Could you check a few things on this drawing? It's one solid part, dimensions in mm from its lowest x, y, z. Give positions to 0.01 mm unless a question says otherwise; leave off trailing zeros. Loops run counter-clockwise (first coordinate to the right, second up) from the corner with the lowest first, then second, coordinate; pieces in that order, holes last.
Q1. Suppose I cut it at B-B (x = 19.05). List the corners of the cut face in (y, z) for me, and give its area (3 significant figures).
Q2. Suppose I cut it at D-D (y = 43.9). List the corners of the cut face in (x, z) for me.
Q3. Suppose I cut it at C-C (z = 1.95). List the corners of the cut face in (x, y) for me, and give its area (3 significant figures).
Q4. Suppose I cut it at A-A (y = 25.4). List the corners of the cut face in (x, z) for me, and give its area (3 significant figures).
Q5. I need wall thicknesses on probe 1 along Y at (x, z) = (19.05, 2.5); probe 2 along X at (y, z) = (25.4, 1.8); probe 3 along X at (y, z) = (6.9, 2.05). Which ranges of each line are inside material? Lowest first, please.
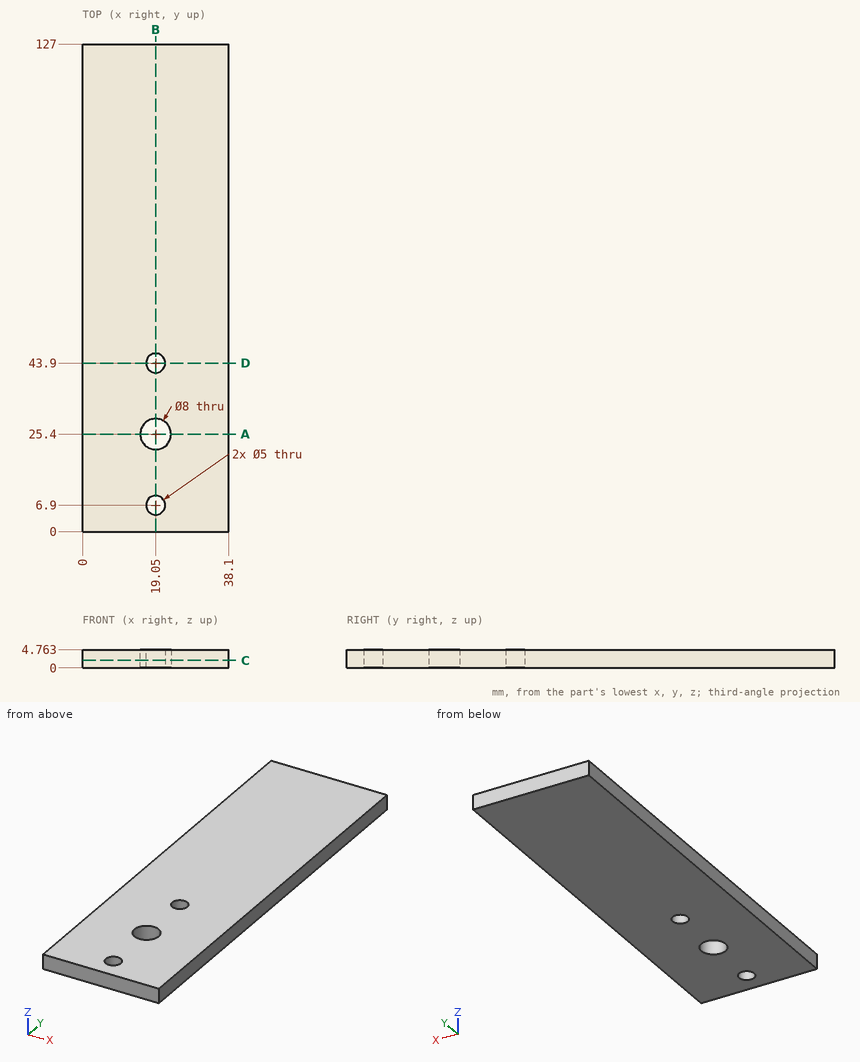
Solutions:
1. outline: (0, 0) - (4.4, 0) - (4.4, 4.76) - (0, 4.76) - close; (9.4, 0) - (21.4, 0) - (21.4, 4.76) - (9.4, 4.76) - close; (29.4, 0) - (41.4, 0) - (41.4, 4.76) - (29.4, 4.76) - close; (46.4, 0) - (127, 0) - (127, 4.76) - (46.4, 4.76) - close
1. area: 519 mm2
2. outline: (0, 0) - (16.55, 0) - (16.55, 4.76) - (0, 4.76) - close; (21.55, 0) - (38.1, 0) - (38.1, 4.76) - (21.55, 4.76) - close
3. outline: (0, 0) - (38.1, 0) - (38.1, 127) - (0, 127) - close; hole circle Ø8 at (19.05, 25.4); hole circle Ø5 at (19.05, 6.9); hole circle Ø5 at (19.05, 43.9)
3. area: 4,750 mm2
4. outline: (0, 0) - (15.05, 0) - (15.05, 4.76) - (0, 4.76) - close; (23.05, 0) - (38.1, 0) - (38.1, 4.76) - (23.05, 4.76) - close
4. area: 143 mm2
5. probe 1: y = 0 to 4.4, 9.4 to 21.4, 29.4 to 41.4, 46.4 to 127
5. probe 2: x = 0 to 15.05, 23.05 to 38.1
5. probe 3: x = 0 to 16.55, 21.55 to 38.1
